```python
from build123d import *

# Parameters (mm, degrees)
F0_W          = 430
F0_H          = 20
F1_DEPTH      = 70
F2_W          = 5
F2_H          = 10
F3_DEPTH      = 415
F3_DEPTH_BACK = 15
F4_W          = 20
F4_H          = 25
F4_H_2        = 20
F5_DEPTH      = 20.001


with BuildPart() as f1:
    # F0 (on Top) → F1 (new body)
    with BuildSketch(Plane.XY):
        with Locations((-189.742246, -17.948127)):
            Rectangle(F0_W, F0_H)
    extrude(amount=F1_DEPTH)

    # F2 (on face) → F3 (cut, two sides)
    with BuildSketch(Plane.YZ.offset(25.257754)) as f3_sk:
        with Locations((-25.448127, 55)):
            Rectangle(F2_W, F2_H)
    extrude(amount=-F3_DEPTH, mode=Mode.SUBTRACT)
    extrude(f3_sk.sketch, amount=-F3_DEPTH_BACK, mode=Mode.SUBTRACT)

    # F4 (on face) → F5 (cut, through all)
    with BuildSketch(Plane(origin=(0, -7.948127, 0), x_dir=(-1, 0, 0), z_dir=(0, 1, 0))):
        with Locations((-15.257754, 57.5)):
            Rectangle(F4_W, F4_H)
        with Locations((-15.257754, 12.5)):
            Rectangle(F4_W, F4_H)
        with Locations((394.742246, 35)):
            Rectangle(F4_W, F4_H_2)
    extrude(amount=-F5_DEPTH, mode=Mode.SUBTRACT)


solid = f1.part
```
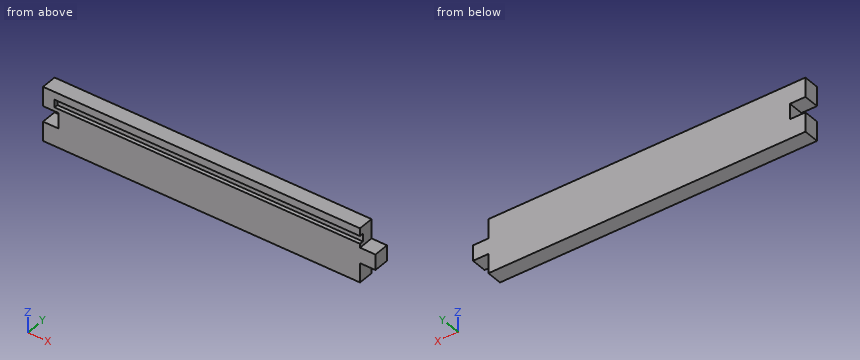
Input: part model. Units: mm. Frame: model coordinates. Round coordinates to 2 decimals unless told otherwise and drop trailing zeros. Loops run counter-clockwise (first coordinate to the right, second up) from the corner with the lowest first, then second, coordinate; pieces in that order, holes last. Notation, with made-up numbers: (-18.5, 47.5) -> (18.5, 47.5) arc R23 cw to (18.5, 61.5) -> close; hole circle Ø11 at (45.25, -25). An arc over 180 degrees is marked (long way). One line per item, written item: value.
(1) Pin query (flat end, axial travel): pin 1 (6 mm diameter, centred on x = 14, y = -20.5, fed in from -Z); pin 2 (10 mm diameter, centred on x = -297, y = -21, fed in from -Z); pin 3 (10 mm diameter, centred on x = 17.5, y = -21.5, fed in from +Z); pin 4 (2 mm diameter, centred on y = -14.5, z = 58, fed in from +X). Return the tip coordinate at first contact, or that it passes through.
Geometry check:
pin 1: z = 25
pin 2: z = 0
pin 3: z = 45
pin 4: x = 5.26
(2) Section A-A (x = -187). Return the cut outline in (y, z), plus the area to 3 significant figures.
Geometry check:
outline: (-27.95, 0) -> (-7.95, 0) -> (-7.95, 70) -> (-27.95, 70) -> (-27.95, 60) -> (-22.95, 60) -> (-22.95, 50) -> (-27.95, 50) -> close
area: 1,350 mm2
(3) Material intervals for line 1 (Z direction, x = -49.5, y = -27); line 2 (X direction, y = -11.75, z = 3.5); line 3 (X direction, y = -22.25, z = 36), sorted ascending. Write a range as [from, to].
Geometry check:
line 1: [0, 50], [60, 70]
line 2: [-404.74, 5.26]
line 3: [-384.74, 25.26]
(4) Section D-D (z = 14.5). Return the cut outline in (x, y).
Geometry check:
outline: (-404.74, -27.95) -> (5.26, -27.95) -> (5.26, -7.95) -> (-404.74, -7.95) -> close
(5) Section C-C (z = 56.5). Return the cut outline in (x, y), plus the area to 4 significant figures.
Geometry check:
outline: (-404.74, -27.95) -> (-389.74, -27.95) -> (-389.74, -22.95) -> (5.26, -22.95) -> (5.26, -7.95) -> (-404.74, -7.95) -> close
area: 6,225 mm2
(6) Section B-B (y = -15.25). Return the cut outline in (x, z), plus the area to 3 significant figures.
Geometry check:
outline: (-404.74, 0) -> (5.26, 0) -> (5.26, 25) -> (25.26, 25) -> (25.26, 45) -> (5.26, 45) -> (5.26, 70) -> (-404.74, 70) -> (-404.74, 45) -> (-384.74, 45) -> (-384.74, 25) -> (-404.74, 25) -> close
area: 28,700 mm2
